Input: part model. Units: mm. Frame: model coordinates. Face numbers are marked on the shaded views. A direction names the side the tool comes from. Round coordinates to 2 decimals unless told otherwise and drop trailing zeros. Loops run counter-clockwise (first coordinate to the right, second up) from the corner with the lowest first, then second, coordinate; pieces in that order, holes last. Notation, with made-up numbers: (87.5, 70.5) -> (146.5, 70.5) arc R15 cw to (146.5, 89.5) -> close; hole circle Ø6 at (60.25, 56). An arc over 180 degrees is marked (long way). Answer as a JSON object with one key per item and string values. Group by question number.
Item 1: Material intervals for line 1 (Z direction, x = 8, y = -3.5); line 2 (Y direction, x = -0.25, z = -55); line 3 (Z direction, x = 1.25, y = -6.5), sorted ascending. Write a range as [from, to].
Item 2: Section query D-D on x = 1. Return loops of the section in (y, z), and give its area (3 significant figures).
Item 3: Section query C-C on z = -28. Return loops of the section in (x, y), and give its area (3 significant figures).
Item 4: Section query A-A on y = 0. Return loops of the section in (x, z), and give its area (3 significant figures).
Item 5: Set-up query: the marked faces 1, 2, 3, 4 and 5. Return all of +Z, -Z, +X, -X, +Y, -Y with unobstructed straight access to the full face (end or side cutting, diameter ignored); none if empty.
Item 6: Section query B-B on x = -5.25. Return loops of the section in (y, z), and give its area (3 significant figures).
Item 7: Pin query (flat end, axial travel): pin 1 (2.5 mm diameter, centred on y = -1.5, z = 4, fed in from +X); pin 2 (1.5 mm diameter, centred on x = -4, y = 6, fed in from -Z); pin 3 (10 mm diameter, centred on x = -5, y = 1.5, fed in from -Z); pin 4 (6 mm diameter, centred on y = 2.5, z = -37.5, fed in from -X). Return the tip coordinate at first contact, or that it passes through.
from build123d import *

# Parameters (mm, degrees)
EXTRUDE_SKETCH_1_R = 9.06
EXTRUDE_1_DEPTH    = 1.44
EXTRUDE_START      = 1.44
EXTRUDE_2_DEPTH    = 5.2
EXTRUDE_START_2    = -60
EXTRUDE_SKETCH_3_R = 4
EXTRUDE_3_DEPTH    = 60.01


with BuildPart() as part:
    # Extrude sketch 1 → Extrude 1 (new body)
    with BuildSketch(Plane.XY):
        with Locations(Location((0, 0, 0), (0, 0, 180))):
            Circle(EXTRUDE_SKETCH_1_R)
    extrude(amount=EXTRUDE_1_DEPTH)


with BuildPart() as body_2:
    # Extrude sketch 2 → Extrude 2 (new body)
    with BuildSketch(Plane.XY.offset(EXTRUDE_START)):
        Polygon((6.5, 3.75277675), (0, 7.505553499), (-6.5, 3.75277675), (-6.5, -3.75277675), (0, -7.505553499), (6.5, -3.75277675), align=None)
    extrude(amount=EXTRUDE_2_DEPTH)


with BuildPart() as body_3:
    # Extrude sketch 3 → Extrude 3 (new body)
    with BuildSketch(Plane.XY.offset(EXTRUDE_START_2)):
        with Locations(Location((0, 0, 0), (0, 0, 180))):
            Circle(EXTRUDE_SKETCH_3_R)
    extrude(amount=EXTRUDE_3_DEPTH)


with BuildPart() as body_2_1:
    add(body_2.part)

    # Combine _weld _ assembly of features: union part, body 3
    add(part.part)
    add(body_3.part)


solid = body_2_1.part
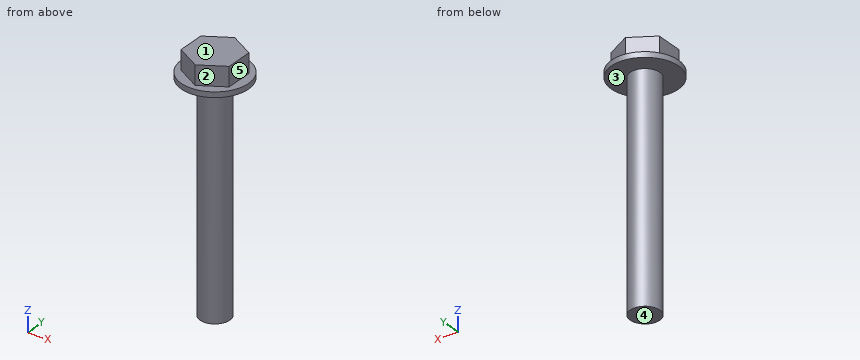
Solved:
{
 "1": {"line 1": "[0, 1.44]", "line 2": "[-3.99, 3.99]", "line 3": "[0, 6.64]"},
 "2": {"outline": "(-9, 0) -> (-3.87, 0) -> (-3.87, -60) -> (3.87, -60) -> (3.87, 0) -> (9, 0) -> (9, 1.44) -> (6.93, 1.44) -> (6.93, 6.64) -> (-6.93, 6.64) -> (-6.93, 1.44) -> (-9, 1.44) -> close", "area": "563 mm²"},
 "3": {"outline": "circle Ø8 at (0, 0)", "area": "50.3 mm²"},
 "4": {"outline": "(-9.06, 0) -> (-4, 0) -> (-4, -60) -> (4, -60) -> (4, 0) -> (9.06, 0) -> (9.06, 1.44) -> (6.5, 1.44) -> (6.5, 6.64) -> (-6.5, 6.64) -> (-6.5, 1.44) -> (-9.06, 1.44) -> close", "area": "574 mm²"},
 "5": {"face 1": "+Z, +X, -X, +Y, -Y", "face 2": "+Z, +X, -Y", "face 3": "-Z", "face 4": "-Z, +X, -X, +Y, -Y", "face 5": "+Z, +X, +Y, -Y"},
 "6": {"outline": "(-7.38, 0) -> (7.38, 0) -> (7.38, 1.44) -> (4.47, 1.44) -> (4.47, 6.64) -> (-4.47, 6.64) -> (-4.47, 1.44) -> (-7.38, 1.44) -> close", "area": "67.8 mm²"},
 "7": {"pin 1": "x = 6.5", "pin 2": "z = 0", "pin 3": "z = -60", "pin 4": "x = -4"}
}
